Part model, mm, in its own coordinate system. Face numbers are marked on the shaded views. A direction names the side the tool comes from. Coordinates: 2 decimals unless noted, no trailing zeros. Loops run counter-clockwise (first coordinate to the right, second up) from the corner with the lowest first, then second, coordinate; pieces in that order, holes last. Notation, with made-up numbers: (7.25, 31.25) -> (61.25, 31.25) arc R15 ccw to (61.25, 41.25) -> close; hole circle Ø6 at (-33.5, 50.5). An arc over 180 degrees is marked (long way). One line per question, with ' | ' between items. Start each with the question number.
1) Probe L1, parallel to X at y = -28, z = 8.5; L2, parallel to Y at x = -21, z = 9; L3, parallel to Y at x = -22.5, z = 9. List the from-to ranges inside material, lowest first. Write a range as from..to.
2) 3-axis set-ups, long thin cutter, end or side, ignore diameter. For the marked faces 1 and 2: which of +Z, -Z, +X, -X, +Y, -Y reach the whole face in a straight line?
3) Drop flat-ended pins along their axis: pin 1 (6 mm diameter, centred on x = -22.5, z = 12, fed in from +Y); pin 2 (1 mm diameter, centred on x = 2, z = 16, fed in from +Y); pin 3 (2.5 mm diameter, centred on y = 30, z = 10, fed in from -X). Give the stop position or say it passes through.
4) Cut at B-B (y = -23). List the corners of the cut face in (x, z).
5) Cut at A-A (z = 9). Count the separate pieces of the cut face and the enclosed holes in it, plus the area to 3 significant figures.
6) Two-plate mould, pull along X, no slides. Class the marked faces 3, 4, 5 and 6: released by +X, released by -X, zero draft, split by the parting line, or undercut.
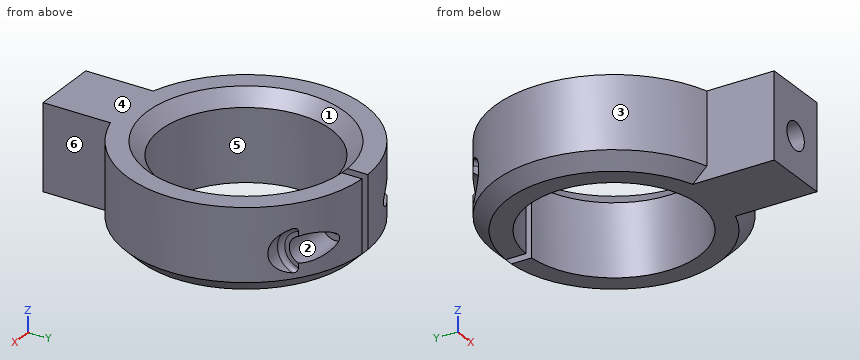
from build123d import *

# Parameters (mm, degrees)
BOSS_EXTRUDE1_DEPTH     = 16
SKETCH2_R               = 3.05
CUT_EXTRUDE1_DEPTH      = 15
BOSS_EXTRUDE2_DEPTH     = 3
CHAMFER4_SIZE           = 3
CUT_EXTRUDE2_DEPTH      = 29
CUT_EXTRUDE2_DEPTH_BACK = 25
SKETCH4_R               = 1.5
SKETCH5_R               = 2.5
CUT_EXTRUDE3_DEPTH      = 27.5
SKETCH6_R               = 3
CUT_EXTRUDE4_DEPTH      = 22.5
SKETCH5_3_R             = 5
SKETCH5_3_R_2           = 2.5
CUT_EXTRUDE5_DEPTH      = 11
SKETCH6_3_R             = 5
SKETCH6_3_R_2           = 3
CUT_EXTRUDE6_DEPTH      = 11
FILLET1_R               = 1


with BuildPart() as part:
    # Sketch1 → Boss-Extrude1 (new body)
    with BuildSketch(Plane.XY):
        with BuildLine():
            ThreePointArc((-14.719179189, 28.233250262), (-15.719179189, -9.740415699), (-16.719179189, 28.233250262))
            Line((-16.719179189, 28.233250262), (-16.719179189, 35.740709655))
            ThreePointArc((-16.719179189, 35.740709655), (-42.013744392, 12.552886715), (-23.219179189, -16.156945753))
            Line((-23.219179189, -16.156945753), (-23.219179189, -31.156945753))
            Line((-23.219179189, -31.156945753), (-8.219179189, -31.156945753))
            Line((-8.219179189, -31.156945753), (-8.219179189, -16.156945753))
            ThreePointArc((-8.219179189, -16.156945753), (10.575386014, 12.552886715), (-14.719179189, 35.740709655))
            Line((-14.719179189, 35.740709655), (-14.719179189, 28.233250262))
        make_face()
    extrude(amount=BOSS_EXTRUDE1_DEPTH)

    # Sketch2 → Cut-Extrude1 (cut)
    with BuildSketch(Plane.XZ.offset(31.156945753)):
        with Locations(Location((-15.719179189, 8.5, 0), (0, 0, 270))):
            Circle(SKETCH2_R)
    extrude(amount=-CUT_EXTRUDE1_DEPTH, mode=Mode.SUBTRACT)

    # Sketch3 → Boss-Extrude2 (add)
    with BuildSketch(Plane.XY.offset(16)):
        with BuildLine():
            ThreePointArc((-14.719179189, 28.233250262), (-15.719179189, -9.740415699), (-16.719179189, 28.233250262))
            Line((-16.719179189, 28.233250262), (-16.719179189, 35.740709655))
            ThreePointArc((-16.719179189, 35.740709655), (-42.013744392, 12.552886715), (-23.219179189, -16.156945753))
            Line((-23.219179189, -16.156945753), (-23.219179189, -31.156945753))
            Line((-23.219179189, -31.156945753), (-8.219179189, -31.156945753))
            Line((-8.219179189, -31.156945753), (-8.219179189, -16.156945753))
            ThreePointArc((-8.219179189, -16.156945753), (10.575386014, 12.552886715), (-14.719179189, 35.740709655))
            Line((-14.719179189, 35.740709655), (-14.719179189, 28.233250262))
        make_face()
    extrude(amount=BOSS_EXTRUDE2_DEPTH)

    # Chamfer4
    chamfer4_edges = [part.edges().sort_by_distance(p)[0] for p in [
        (-15.719179189, -9.740415699, 19),
        (10.575386014, 12.552886715, 0),
        (-42.013744392, 12.552886715, 0),
    ]]
    chamfer(chamfer4_edges, length=CHAMFER4_SIZE)

    # Sketch4 → Cut-Extrude2 (cut, two sides: drawn at the far end of the back side and taken through both)
    with BuildSketch(Plane.ZY.offset(14.719179189).offset(-CUT_EXTRUDE2_DEPTH_BACK)):
        with Locations(Location((9, 31.740709655, 0), (0, 0, 180))):
            Circle(SKETCH4_R)
    extrude(amount=CUT_EXTRUDE2_DEPTH + CUT_EXTRUDE2_DEPTH_BACK, mode=Mode.SUBTRACT)

    # Sketch5 → Cut-Extrude3 (cut)
    with BuildSketch(Plane.ZY.offset(42.219179189)):
        with Locations((9, 31.740709655)):
            Circle(SKETCH5_R)
    extrude(amount=-CUT_EXTRUDE3_DEPTH, mode=Mode.SUBTRACT)

    # Sketch6 → Cut-Extrude4 (cut)
    with BuildSketch(Plane(origin=(10.780820811, 0, 0), x_dir=(0, 0, -1), z_dir=(1, 0, 0))):
        with Locations((-9, 31.740709655)):
            Circle(SKETCH6_R)
    extrude(amount=-CUT_EXTRUDE4_DEPTH, mode=Mode.SUBTRACT)

    # Sketch5<3> → Cut-Extrude5 (cut)
    with BuildSketch(Plane.ZY.offset(42.219179189)):
        with Locations((9, 31.740709655)):
            Circle(SKETCH5_3_R)
        with Locations(Location((9, 31.740709655, 0), (0, 0, 336.747995985))):
            Circle(SKETCH5_3_R_2, mode=Mode.SUBTRACT)
    extrude(amount=-CUT_EXTRUDE5_DEPTH, mode=Mode.SUBTRACT)

    # Sketch6<3> → Cut-Extrude6 (cut)
    with BuildSketch(Plane(origin=(10.780820811, 0, 0), x_dir=(0, 0, -1), z_dir=(1, 0, 0))):
        with Locations((-9, 31.740709655)):
            Circle(SKETCH6_3_R)
        with Locations(Location((-9, 31.740709655, 0), (0, 0, 340.793122324))):
            Circle(SKETCH6_3_R_2, mode=Mode.SUBTRACT)
    extrude(amount=-CUT_EXTRUDE6_DEPTH, mode=Mode.SUBTRACT)

    # Fillet1
    fillet1_edges = [part.edges().sort_by_distance(p)[0] for p in [
        (-31.219179189, 26.740709655, 9),
        (-0.219179189, 26.740709655, 9),
    ]]
    fillet(fillet1_edges, radius=FILLET1_R)


solid = part.part
Reported:
1) L1: x = -23.22..-18.77, -12.67..-8.22 | L2: y = -31.16..-8.99, 27.51..29.24, 34.24..35.23 | L3: y = -31.16..-8.49, 27.01..29.24, 34.24..34.88
2) face 1: +Z | face 2: +X
3) pin 1: stops at y = 35.49 | pin 2: stops at y = 29.4 | pin 3: stops at x = -31.22
4) outline: (-23.22, 0) -> (-8.22, 0) -> (-8.22, 19) -> (-23.22, 19) -> close; hole circle Ø6.1 at (-15.72, 8.5)
5) separate pieces: 3 | enclosed holes: 0 | area: 1,040 mm²
6) face 3: released by -X | face 4: zero draft | face 5: undercut | face 6: released by +X
